For this review, use the dimensioned drawing (mm, ordinates from the lowest corner) and the shaded views. A direction names the side the tool comes from. Give positions to 0.01 mm unless a question says otherwise; leave off trailing zeros. Write each loop counter-clockwise with the first axis right and the second up, starting at its lowest first coordinate (ties: lowest second). Pieces come first, ordered by that corner, then holes. Notation, with made-up numbers: (-19, 51.25) - (34, 51.25) arc R23 cw to (34, 80.25) - close; hole circle Ø2 at (11.25, 53). An arc over 180 degrees is marked (long way). Use a Markdown table: item, result. Add a question column.
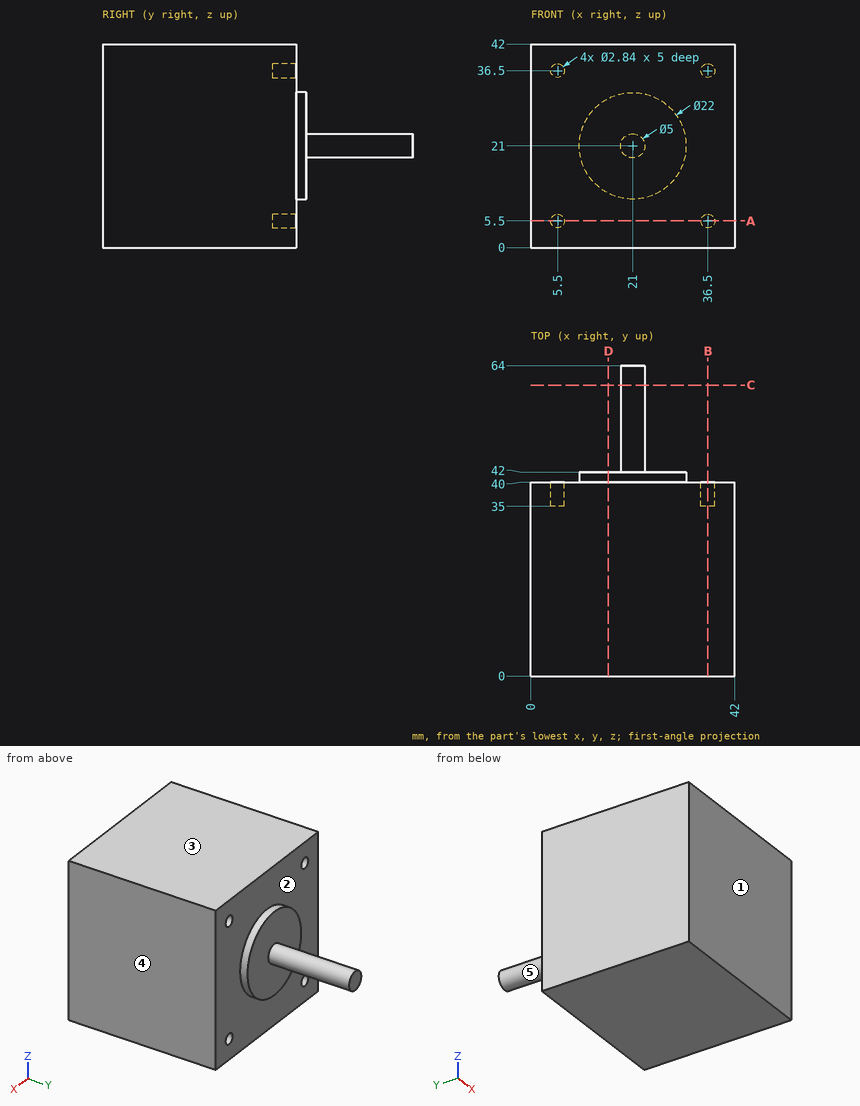
(1) Add section D-D (x = 16). State the section outline as (y, z) points.
(2) Add section C-C (y = 60). State the section outline as (x, z) points, and give its area (3 significant figures).
(3) Tool access review of the marked faces 4 and 5: name each direction out of +Z, -Z, +X, -X, +Y, -Y from which nothing blocks a thin tool from reaching the whole face with its end or side.
(4) Add section B-B (x = 36.5). State the section outline as (y, z) points.
(5) Mouldability with a two-part tool opening along Y and no side actions: class the marked faces 1, 2 and 3 as +Y half, -Y half, draft (parallel to the pull), parting line (faces both ways), or undercut.
(6) Add section A-A (z = 5.5). State the section outline as (x, y) points.
(7) For line 1 along Z through (x, y) = (36.5, 38.35); line 2 along Z through (x, y) = (36, 37), list the stretches that pass through material, from the lowest coordinate up.
(8) Insertion check: pin 1 (0.9 mm diameter, centred on x = 5.5, z = 37, fed in from +Y); pin 2 (3.5 mm diameter, centred on x = 5.5, z = 5.5, fed in from +Y). Each pin has a flat end and moves straight along its axis. Give the tip position at first contact, or say it passes through.
Answers follow:
| question | item | result |
|---|---|---|
| 1 | outline | (0, 0) - (40, 0) - (40, 11.2) - (42, 11.2) - (42, 30.8) - (40, 30.8) - (40, 42) - (0, 42) - close |
| 2 | outline | circle Ø5 at (21, 21) |
| 2 | area | 19.6 mm^2 |
| 3 | face 4 | +Z, -Z, +X, +Y, -Y |
| 3 | face 5 | +Y |
| 4 | outline | (0, 0) - (40, 0) - (40, 4.08) - (35, 4.08) - (35, 6.92) - (40, 6.92) - (40, 35.08) - (35, 35.08) - (35, 37.92) - (40, 37.92) - (40, 42) - (0, 42) - close |
| 5 | face 1 | -Y half |
| 5 | face 2 | +Y half |
| 5 | face 3 | draft |
| 6 | outline | (0, 0) - (42, 0) - (42, 40) - (37.92, 40) - (37.92, 35) - (35.08, 35) - (35.08, 40) - (6.92, 40) - (6.92, 35) - (4.08, 35) - (4.08, 40) - (0, 40) - close |
| 7 | line 1 | 0 to 4.08, 6.92 to 35.08, 37.92 to 42 |
| 7 | line 2 | 0 to 4.17, 6.83 to 35.17, 37.83 to 42 |
| 8 | pin 1 | y = 35 |
| 8 | pin 2 | y = 40 |
